Check sheet for the drawn part. Datum: minimum x, y, z corner. Units: mm. A direction names the side the tool comes from. Give positions to 0.01 mm unless a question says otherwise; leave off trailing zeros. Write each loop counter-clockwise with the first axis right and the second up, starting at its lowest first coordinate (ties: lowest second). Pieces come first, ordered by that corner, then holes. Notation, with made-up numbers: M -10,63.5 L 20,63.5 A9 ccw 20,67.5 Z; hole C 3,61 d11. An arc over 180 degrees is marked long. Write item = value, one per line. Start each with the question number.
1) Scan lines: L1, parallel to Z at x = 30, y = 51; L2, parallel to X at y = 10, z = 25.5; L3, parallel to Y at x = 21.5, z = 12. Record each from-to range of solid material in increasing order.
2) Sectioned sample at A-A, the plane z = 31. Record the cut outline in (x, y), then the cut area to 3 significant figures.
3) Set-up check for the marked faces 1 and 2: record each of +Z, -Z, +X, -X, +Y, -Y from which the full face is reachable in a straight line by a thin tool's end or side.
4) Sectioned sample at B-B, the plane x = 42.5. Record the cut outline in (y, z).
5) Gauge pin test, flat ends, axial feed: pin 1 (4 mm diameter, centred on y = 38.5, z = 43, fed in from +X); pin 2 (8 mm diameter, centred on x = 24.5, y = 34, fed in from -Z); pin 3 (7 mm diameter, centred on x = 52.31, z = 11.25, fed in from +Y). Record the tip position at first contact, or that the pin passes through.
6) Sectioned sample at C-C, the plane z = 46. Count the separate pieces of the cut face and the enclosed holes in it.
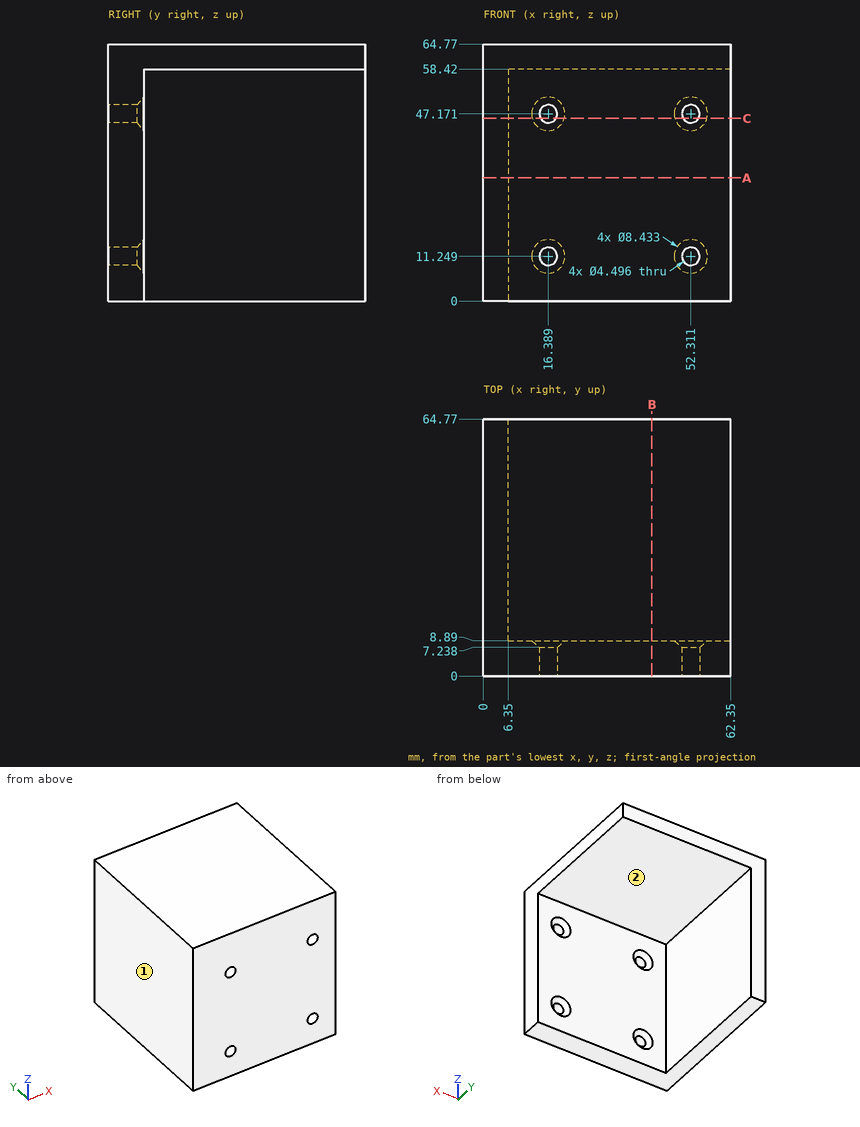
Data:
q1.L1 = 58.42 to 64.77
q1.L2 = 0 to 6.35
q1.L3 = 0 to 8.89
q2.outline = M 0,0 L 62.35,0 L 62.35,8.89 L 6.35,8.89 L 6.35,64.77 L 0,64.77 Z
q2.area = 909 mm2
q3.face_1 = +Z, -Z, -X, +Y, -Y
q3.face_2 = -Z, +X, +Y
q4.outline = M 0,0 L 8.89,0 L 8.89,58.42 L 64.77,58.42 L 64.77,64.77 L 0,64.77 Z
q5.pin_1 = 6.35
q5.pin_2 = 58.42
q5.pin_3 = 8.29
q6.separate_pieces = 3
q6.enclosed_holes = 0
